```python
from build123d import *

# Parameters (mm, degrees)
F1_DEPTH = 200


with BuildPart() as f1:
    # F0 (on Front) → F1 (new body)
    with BuildSketch(Plane.XZ):
        with BuildLine():
            Line((0, 41.25), (0, 44.5))
            Line((0, 44.5), (-9.5, 44.5))
            Line((-9.5, 44.5), (-9.5, 45))
            Line((-9.5, 45), (-17, 45))
            Line((-17, 45), (-17, 44.5))
            Line((-17, 44.5), (-17.5, 44.5))
            Line((-17.5, 44.5), (-17.5, 39))
            Line((-17.5, 39), (-12.5, 39))
            Line((-12.5, 39), (-12.5, 32))
            Line((-12.5, 32), (-29.5, 32))
            Line((-29.5, 32), (-33.5, 36))
            Line((-33.5, 36), (-33.5, 39))
            Line((-33.5, 39), (-27.5, 39))
            Line((-27.5, 39), (-27.5, 44.5))
            Line((-27.5, 44.5), (-28, 44.5))
            Line((-28, 44.5), (-28, 45))
            Line((-28, 45), (-40, 45))
            ThreePointArc((-40, 45), (-43.535534, 43.535534), (-45, 40))
            Line((-45, 40), (-45, 28))
            Line((-45, 28), (-44.5, 28))
            Line((-44.5, 28), (-44.5, 27.5))
            Line((-44.5, 27.5), (-39, 27.5))
            Line((-39, 27.5), (-39, 33.5))
            Line((-39, 33.5), (-36, 33.5))
            Line((-36, 33.5), (-32, 29.5))
            Line((-32, 29.5), (-32, 12.5))
            Line((-32, 12.5), (-39, 12.5))
            Line((-39, 12.5), (-39, 17.5))
            Line((-39, 17.5), (-44.5, 17.5))
            Line((-44.5, 17.5), (-44.5, 17))
            Line((-44.5, 17), (-45, 17))
            Line((-45, 17), (-45, 9.5))
            Line((-45, 9.5), (-44.5, 9.5))
            Line((-44.5, 9.5), (-44.5, 0))
            Line((-44.5, 0), (-41.25, 0))
            ThreePointArc((-41.25, 0), (-36.25, 5), (-31.25, 0))
            Line((-31.25, 0), (-28, 0))
            Line((-28, 0), (-28, 25.5))
            Line((-28, 25.5), (-12, 9.5))
            Line((-12, 9.5), (-12, 0))
            Line((-12, 0), (-7.5, 0))
            ThreePointArc((-7.5, 0), (-5.303301, 5.303301), (0, 7.5))
            Line((0, 7.5), (0, 12))
            Line((0, 12), (-9.5, 12))
            Line((-9.5, 12), (-25.5, 28))
            Line((-25.5, 28), (0, 28))
            Line((0, 28), (0, 31.25))
            ThreePointArc((0, 31.25), (-5, 36.25), (0, 41.25))
        make_face()
        with BuildLine():
            Line((40, 45), (28, 45))
            Line((28, 45), (28, 44.5))
            Line((28, 44.5), (27.5, 44.5))
            Line((27.5, 44.5), (27.5, 39))
            Line((27.5, 39), (33.5, 39))
            Line((33.5, 39), (33.5, 36))
            Line((33.5, 36), (29.5, 32))
            Line((29.5, 32), (12.5, 32))
            Line((12.5, 32), (12.5, 39))
            Line((12.5, 39), (17.5, 39))
            Line((17.5, 39), (17.5, 44.5))
            Line((17.5, 44.5), (17, 44.5))
            Line((17, 44.5), (17, 45))
            Line((17, 45), (9.5, 45))
            Line((9.5, 45), (9.5, 44.5))
            Line((9.5, 44.5), (0, 44.5))
            Line((0, 44.5), (0, 41.25))
            ThreePointArc((0, 41.25), (5, 36.25), (0, 31.25))
            Line((0, 31.25), (0, 28))
            Line((0, 28), (25.5, 28))
            Line((25.5, 28), (9.5, 12))
            Line((9.5, 12), (0, 12))
            Line((0, 12), (0, 7.5))
            ThreePointArc((0, 7.5), (5.303301, 5.303301), (7.5, 0))
            Line((7.5, 0), (12, 0))
            Line((12, 0), (12, 9.5))
            Line((12, 9.5), (28, 25.5))
            Line((28, 25.5), (28, 0))
            Line((28, 0), (31.25, 0))
            ThreePointArc((31.25, 0), (36.25, 5), (41.25, 0))
            Line((41.25, 0), (44.5, 0))
            Line((44.5, 0), (44.5, 9.5))
            Line((44.5, 9.5), (45, 9.5))
            Line((45, 9.5), (45, 17))
            Line((45, 17), (44.5, 17))
            Line((44.5, 17), (44.5, 17.5))
            Line((44.5, 17.5), (39, 17.5))
            Line((39, 17.5), (39, 12.5))
            Line((39, 12.5), (32, 12.5))
            Line((32, 12.5), (32, 29.5))
            Line((32, 29.5), (36, 33.5))
            Line((36, 33.5), (39, 33.5))
            Line((39, 33.5), (39, 27.5))
            Line((39, 27.5), (44.5, 27.5))
            Line((44.5, 27.5), (44.5, 28))
            Line((44.5, 28), (45, 28))
            Line((45, 28), (45, 40))
            ThreePointArc((45, 40), (43.535534, 43.535534), (40, 45))
        make_face()
        with BuildLine():
            ThreePointArc((0, -7.5), (-5.303301, -5.303301), (-7.5, 0))
            Line((-7.5, 0), (-12, 0))
            Line((-12, 0), (-12, -9.5))
            Line((-12, -9.5), (-28, -25.5))
            Line((-28, -25.5), (-28, 0))
            Line((-28, 0), (-31.25, 0))
            ThreePointArc((-31.25, 0), (-36.25, -5), (-41.25, 0))
            Line((-41.25, 0), (-44.5, 0))
            Line((-44.5, 0), (-44.5, -9.5))
            Line((-44.5, -9.5), (-45, -9.5))
            Line((-45, -9.5), (-45, -17))
            Line((-45, -17), (-44.5, -17))
            Line((-44.5, -17), (-44.5, -17.5))
            Line((-44.5, -17.5), (-39, -17.5))
            Line((-39, -17.5), (-39, -12.5))
            Line((-39, -12.5), (-32, -12.5))
            Line((-32, -12.5), (-32, -29.5))
            Line((-32, -29.5), (-36, -33.5))
            Line((-36, -33.5), (-39, -33.5))
            Line((-39, -33.5), (-39, -27.5))
            Line((-39, -27.5), (-44.5, -27.5))
            Line((-44.5, -27.5), (-44.5, -28))
            Line((-44.5, -28), (-45, -28))
            Line((-45, -28), (-45, -40))
            ThreePointArc((-45, -40), (-43.535534, -43.535534), (-40, -45))
            Line((-40, -45), (-28, -45))
            Line((-28, -45), (-28, -44.5))
            Line((-28, -44.5), (-27.5, -44.5))
            Line((-27.5, -44.5), (-27.5, -39))
            Line((-27.5, -39), (-33.5, -39))
            Line((-33.5, -39), (-33.5, -36))
            Line((-33.5, -36), (-29.5, -32))
            Line((-29.5, -32), (-12.5, -32))
            Line((-12.5, -32), (-12.5, -39))
            Line((-12.5, -39), (-17.5, -39))
            Line((-17.5, -39), (-17.5, -44.5))
            Line((-17.5, -44.5), (-17, -44.5))
            Line((-17, -44.5), (-17, -45))
            Line((-17, -45), (-9.5, -45))
            Line((-9.5, -45), (-9.5, -44.5))
            Line((-9.5, -44.5), (0, -44.5))
            Line((0, -44.5), (0, -41.25))
            ThreePointArc((0, -41.25), (-5, -36.25), (0, -31.25))
            Line((0, -31.25), (0, -28))
            Line((0, -28), (-25.5, -28))
            Line((-25.5, -28), (-9.5, -12))
            Line((-9.5, -12), (0, -12))
            Line((0, -12), (0, -7.5))
        make_face()
        with BuildLine():
            Line((44.5, -9.5), (44.5, 0))
            Line((44.5, 0), (41.25, 0))
            ThreePointArc((41.25, 0), (36.25, -5), (31.25, 0))
            Line((31.25, 0), (28, 0))
            Line((28, 0), (28, -25.5))
            Line((28, -25.5), (12, -9.5))
            Line((12, -9.5), (12, 0))
            Line((12, 0), (7.5, 0))
            ThreePointArc((7.5, 0), (5.303301, -5.303301), (0, -7.5))
            Line((0, -7.5), (0, -12))
            Line((0, -12), (9.5, -12))
            Line((9.5, -12), (25.5, -28))
            Line((25.5, -28), (0, -28))
            Line((0, -28), (0, -31.25))
            ThreePointArc((0, -31.25), (5, -36.25), (0, -41.25))
            Line((0, -41.25), (0, -44.5))
            Line((0, -44.5), (9.5, -44.5))
            Line((9.5, -44.5), (9.5, -45))
            Line((9.5, -45), (17, -45))
            Line((17, -45), (17, -44.5))
            Line((17, -44.5), (17.5, -44.5))
            Line((17.5, -44.5), (17.5, -39))
            Line((17.5, -39), (12.5, -39))
            Line((12.5, -39), (12.5, -32))
            Line((12.5, -32), (29.5, -32))
            Line((29.5, -32), (33.5, -36))
            Line((33.5, -36), (33.5, -39))
            Line((33.5, -39), (27.5, -39))
            Line((27.5, -39), (27.5, -44.5))
            Line((27.5, -44.5), (28, -44.5))
            Line((28, -44.5), (28, -45))
            Line((28, -45), (40, -45))
            ThreePointArc((40, -45), (43.535534, -43.535534), (45, -40))
            Line((45, -40), (45, -28))
            Line((45, -28), (44.5, -28))
            Line((44.5, -28), (44.5, -27.5))
            Line((44.5, -27.5), (39, -27.5))
            Line((39, -27.5), (39, -33.5))
            Line((39, -33.5), (36, -33.5))
            Line((36, -33.5), (32, -29.5))
            Line((32, -29.5), (32, -12.5))
            Line((32, -12.5), (39, -12.5))
            Line((39, -12.5), (39, -17.5))
            Line((39, -17.5), (44.5, -17.5))
            Line((44.5, -17.5), (44.5, -17))
            Line((44.5, -17), (45, -17))
            Line((45, -17), (45, -9.5))
            Line((45, -9.5), (44.5, -9.5))
        make_face()
    extrude(amount=F1_DEPTH)


solid = f1.part
```
Model file for the job. Use its own axes, mm. A direction names the side the tool comes from. Coordinates: 2 decimals unless noted, no trailing zeros. Write each loop counter-clockwise with the first axis right and the second up, starting at its lowest first coordinate (ties: lowest second). Pieces come first, ordered by that corner, then holes. Notation, with made-up numbers: (70.5, 88.25) - (123.5, 88.25) arc R23 ccw to (123.5, 115.25) - close; hole circle Ø11 at (-36.75, 19). An arc over 180 degrees is marked (long way). One line per item, written item: value. Start each with the question number.
1. Mould opens along X. For faces 5 (the flat face through (-45, -99, 34)), 6 (the flat face through (0, -99, 12)), 7 (the flat face through (45, -99, 13)) say: released by +X, released by -X, zero draft, split by the parting line, or undercut.
2. Tool access for faces 1 (the flat face through (-17.5, -99, -42)), 2 (the flat face through (-27.5, -99, 42)), 3 (the flat face through (-34, -98.6, 31.5)), 4 (the flat face through (-34, -99, 45)): list every direction of +Z, -Z, +X, -X, +Y, -Y with a clear straight run to the whole face (end or side of a thin tool).
3. Slice it at B-B (y = -160). Count the separate pieces of the cut face and the enclosed holes in it, plus the area to 3 significant figures.
4. Probe line 1 (X direction, y = -135, z = -36.25); line 2 (X direction, y = -81, z = -0.5); line 3 (Z direction, x = 36, y = -108). List the from-to ranges inside material, lowest first. Write a range as from..to.
5. Slice it at A-A (z = -22.5). Write the cut outline in (x, y).
6. Flat gauge pins, fed straight in: pin 1 (5.5 mm diameter, centred on y = -104.5, z = -3.5, fed in from -X); pin 2 (4 mm diameter, centred on x = 36, z = 28, fed in from -Y); pin 3 (1.5 mm diameter, centred on x = -4, y = -44.5, fed in from -Z). Where does each tip first touch, or does it go through?
Answers below:
1. face 5: released by -X
1. face 6: undercut
1. face 7: released by +X
2. face 1: -Z, +Y, -Y
2. face 2: +Z, +Y, -Y
2. face 3: +Y, -Y
2. face 4: +Z, +X, -X, +Y, -Y
3. separate pieces: 1
3. enclosed holes: 9
3. area: 3,710 mm^2
4. line 1: x = -45..-33.5, -12.5..-5, 5..12.5, 33.5..45
4. line 2: x = -44.5..-41.22, -31.28..-28, -12..-7.48, 7.48..12, 28..31.28, 41.22..44.5
4. line 3: z = -45..-33.5, -12.5..-4.99, 4.99..12.5, 33.5..45
5. outline: (-32, -200) - (-28, -200) - (-28, 0) - (-32, 0) - close; (-25, -200) - (-20, -200) - (-20, 0) - (-25, 0) - close; (20, -200) - (25, -200) - (25, 0) - (20, 0) - close; (28, -200) - (32, -200) - (32, 0) - (28, 0) - close
6. pin 1: stops at x = -44.5
6. pin 2: passes through
6. pin 3: stops at z = -44.5
